Part model, mm, in its own coordinate system. Face numbers are marked on the shaded views. A direction names the side the tool comes from. Round coordinates to 2 decimals unless told otherwise and drop trailing zeros. Loops run counter-clockwise (first coordinate to the right, second up) from the corner with the lowest first, then second, coordinate; pieces in that order, holes last. Notation, with made-up numbers: (-21.5, -12) -> (32.5, -12) arc R28 cw to (32.5, 10) -> close; hole circle Ø4 at (-2.75, 54.25). An arc over 180 degrees is marked (long way). Use a Markdown table: item, result. Add a question column.
Item 1: Two-plate mould, pull along Z, no slides. Class the marked faces 4, 5, 6 and 7: pulls with the +Z half, pulls with the -Z half, needs draft (parallel to the pull), parting line crosses it, or undercut.
Item 2: Cut at B-B, the plane x = 0. List the corners of the cut face in (y, z).
Item 3: Cut at C-C, the plane z = -1. List the corners of the cut face in (x, y).
Item 4: Cut at A-A, the plane y = -6.35. List the corners of the cut face in (x, z), plus the area to 3 significant figures.
Item 5: Which spindle directions (+Z, -Z, +X, -X, +Y, -Y) get a long thin tool onto all of the face, cutting with end or side? Do the marked faces 1, 2 and 3. Say none if no direction does.
Item 6: Flat gauge pins, fed straight in: pin 1 (3 mm diameter, centred on x = 6.5, z = -2.5, fed in from +Y); pin 2 (2 mm diameter, centred on y = -6.35, z = 0, fed in from +X); pin 3 (1.5 mm diameter, centred on x = 1.5, z = 2, fed in from -Y); pin 4 (3 mm diameter, centred on x = -1, z = 6, fed in from +Y). Where does each tip first touch, or does it go through?
Item 7: Probe line 1 (X direction, y = -7.75, z = 6.75); line 2 (Z direction, x = 0, y = 9.4). List the from-to ranges inside material, lowest first. Write a range as [from, to].
Item 8: Cut at D-D, the plane z = 5. List the corners of the cut face in (x, y), plus the area to 3 significant figures.
```python
from build123d import *

# Parameters (mm, degrees)
EXTRUDE_1_DEPTH     = 10
EXTRUDE_2_DEPTH     = 5
SKETCH_2_R          = 3.2
CUT_EXTRUDE_1_DEPTH = 2.6
SKETCH_4_R          = 1
CUT_EXTRUDE_3_DEPTH = 22.474752618
SKETCH_6_R          = 1.75
CUT_EXTRUDE_4_DEPTH = 26.521608492
FILLET_1_R          = 3
CHAMFER_1_SIZE      = 0.6


with BuildPart() as part:
    # ｽｹｯﾁ1 → ﾎﾞｽ - 押し出し1 (new body)
    with BuildSketch(Plane.XY):
        Polygon((-10.25, 11.45), (-10.25, -11.45), (-5.25, -11.45), (-5.25, -1.25), (5.25, -1.25), (5.25, -11.45), (10.25, -11.45), (10.25, 11.45), align=None)
    extrude(amount=EXTRUDE_1_DEPTH)

    # ｽｹｯﾁ5 → ﾎﾞｽ - 押し出し2 (add)
    with BuildSketch(Plane(origin=(0, 0, 0), x_dir=(-1, 0, 0), z_dir=(0, 0, -1))):
        Polygon((-10.25, 3.75), (10.25, 3.75), (10.25, -11.45), (5.25, -11.45), (5.25, -1.25), (-5.25, -1.25), (-5.25, -11.45), (-10.25, -11.45), align=None)
    extrude(amount=EXTRUDE_2_DEPTH)

    # ｽｹｯﾁ2 → ｶｯﾄ - 押し出し1 (cut)
    with BuildSketch(Plane(origin=(0, 11.45, 0), x_dir=(1, 0, 0), z_dir=(0, 1, 0))):
        with Locations(Location((0, -5, 0), (0, 0, 180))):
            Circle(SKETCH_2_R)
    extrude(amount=-CUT_EXTRUDE_1_DEPTH, mode=Mode.SUBTRACT)

    # ｽｹｯﾁ4 → ｶｯﾄ - 押し出し3 (cut, through all)
    with BuildSketch(Plane.XY.offset(10)):
        with Locations((5.25, -1.25)):
            Circle(SKETCH_4_R)
        with Locations((-5.25, -1.25)):
            Circle(SKETCH_4_R)
    extrude(amount=-CUT_EXTRUDE_3_DEPTH, mode=Mode.SUBTRACT)

    # ｽｹｯﾁ6 → ｶｯﾄ - 押し出し4 (cut, through all)
    with BuildSketch(Plane(origin=(10.25, 0, 0), x_dir=(0, 0, -1), z_dir=(1, 0, 0))):
        with Locations(Location((0, -6.35, 0), (0, 0, 90))):
            Circle(SKETCH_6_R)
    extrude(amount=-CUT_EXTRUDE_4_DEPTH, mode=Mode.SUBTRACT)

    # ﾌｨﾚｯﾄ1
    fillet_1_edges = [part.edges().sort_by_distance(p)[0] for p in [
        (10.25, 0, 10),
        (-10.25, 7.6, 0),
        (10.25, 7.6, 0),
        (-10.25, 0, 10),
    ]]
    fillet(fillet_1_edges, radius=FILLET_1_R)

    # 面取り1
    chamfer_1_edges = [part.edges().sort_by_distance(p)[0] for p in [
        (3.2, 11.45, 5),
        (0, 11.45, 0),
        (-10.25, 11.45, 5),
        (0, 11.45, 10),
        (10.25, 11.45, 5),
        (9.371320344, 11.45, 9.121320344),
        (9.371320344, 11.45, 0.878679656),
        (-9.371320344, 11.45, 9.121320344),
        (-9.371320344, 11.45, 0.878679656),
    ]]
    chamfer(chamfer_1_edges, length=CHAMFER_1_SIZE)


solid = part.part
```
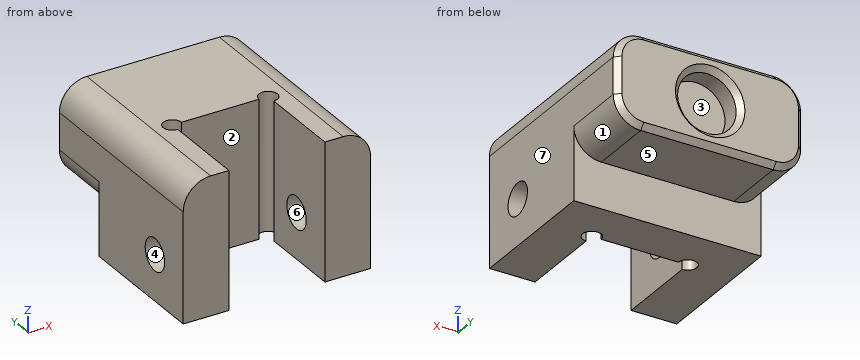
A:
| question | item | result |
|---|---|---|
| 1 | face 4 | undercut |
| 1 | face 5 | pulls with the -Z half |
| 1 | face 6 | undercut |
| 1 | face 7 | needs draft |
| 2 | outline | (-1.25, -5) -> (3.75, -5) -> (3.75, 0) -> (10.85, 0) -> (11.45, 0.6) -> (11.45, 1.2) -> (10.85, 1.8) -> (8.85, 1.8) -> (8.85, 8.2) -> (10.85, 8.2) -> (11.45, 8.8) -> (11.45, 9.4) -> (10.85, 10) -> (-1.25, 10) -> close |
| 3 | outline | (-10.25, -11.45) -> (-5.25, -11.45) -> (-5.25, -7.79) -> (-10.25, -7.79) -> close; (-10.25, -4.91) -> (-5.25, -4.91) -> (-5.25, -2.25) arc R1 cw (long way) to (-4.25, -1.25) -> (4.25, -1.25) arc R1 cw (long way) to (5.25, -2.25) -> (5.25, -4.91) -> (10.25, -4.91) -> (10.25, 3.75) -> (-10.25, 3.75) -> close; (5.25, -11.45) -> (10.25, -11.45) -> (10.25, -7.79) -> (5.25, -7.79) -> close |
| 4 | outline | (-10.25, -5) -> (-5.25, -5) -> (-5.25, -1.75) -> (-10.25, -1.75) -> close; (-10.25, 1.75) -> (-5.25, 1.75) -> (-5.25, 10) -> (-7.25, 10) arc R3 ccw to (-10.25, 7) -> close; (5.25, -5) -> (10.25, -5) -> (10.25, -1.75) -> (5.25, -1.75) -> close; (5.25, 1.75) -> (10.25, 1.75) -> (10.25, 7) arc R3 ccw to (7.25, 10) -> (5.25, 10) -> close |
| 4 | area | 111 mm^2 |
| 5 | face 1 | -Z, +X, +Y |
| 5 | face 2 | +Z, -Z, -Y |
| 5 | face 3 | +Y |
| 6 | pin 1 | stops at y = 3.75 |
| 6 | pin 2 | passes through |
| 6 | pin 3 | stops at y = -1.25 |
| 6 | pin 4 | stops at y = 8.85 |
| 7 | line 1 | x = [-10.25, -5.25], [5.25, 10.25] |
| 7 | line 2 | z = [0, 1.8], [8.2, 10] |
| 8 | outline | (-10.25, -11.45) -> (-5.25, -11.45) -> (-5.25, -2.25) arc R1 cw (long way) to (-4.25, -1.25) -> (4.25, -1.25) arc R1 cw (long way) to (5.25, -2.25) -> (5.25, -11.45) -> (10.25, -11.45) -> (10.25, 10.85) -> (9.65, 11.45) -> (3.8, 11.45) -> (3.2, 10.85) -> (3.2, 8.85) -> (-3.2, 8.85) -> (-3.2, 10.85) -> (-3.8, 11.45) -> (-9.65, 11.45) -> (-10.25, 10.85) -> close |
| 8 | area | 340 mm^2 |
